Read the model definition and answer for the solid it produces. Units are mm, in the model's axes. A direction names the side the tool comes from. Coordinates: 2 decimals unless noted, no trailing zeros. Write each loop counter-clockwise with the first axis right and the second up, starting at its lowest first coordinate (ties: lowest second). Pieces come first, ordered by that corner, then holes.
1) Find the intervals of material crossed by line 1 (Z direction, x = 1774, y = -566.25) (3 decimals); line 2 (Y direction, x = 1786.7, z = 694.25) (3 decimals); line 3 (Z direction, x = 1767.5, y = -562.5) (3 decimals), in increasing order.
2) The part is cut by section A-A (x = 1786.7). Give the number of separate pieces and of enclosed holes in the cut face, then the cut area to 3 significant figures.
3) Each of these flat-tipped pins is pushed along its axis until it touches: pin 1 Ø2 at (x, z) = (1804.5, 580.5) entering from +Y (3 decimals); pin 2 Ø8 at (x, y) = (1775.5, -475.5) entering from -Z (3 decimals); pin 3 Ø11.5 at (x, y) = (1786.7, -480.185) entering from +Z (3 decimals). Where does it stop, or does it pass through?
4) The part is cut by section C-C (z = 425.5). Determine the outline of the cut face in (x, y) (3 decimals).
5) The part is cut by section B-B (y = -457). Determine the outline of the cut face in (x, z) (3 decimals), then the cut area to 3 significant figures.
6) Which of the six approach directions +Z, -Z, +X, -X, +Y, -Y give full straight-line access (tool end or side, diameter ignored) to faces 1 (the face through (1787, -564.085, 500)), 2 (the face through (1784.01, -475.97, 693.12))?
7) Determine the mould class of faces 3 (the face through (1812.1, -568, 501)), 4 (the face through (1782.475, -567.196, 547.743)), 5 (the face through (1787, -507, 696.315)) for opening direction X: +X half, -X half, draft (parallel to the pull), parting line (faces both ways), or undercut.
from build123d import *

# Parameters (mm, degrees)
CROQUIS2_W              = 50.8
CROQUIS2_H              = 6.31
CROQUIS3_W              = 50.8
CROQUIS3_H              = 6.31
CROQUIS4_W              = 60
CROQUIS4_H              = 53.155
SALIENTE_EXTRUIR1_DEPTH = 6.31
CROQUIS5_W              = 60
CROQUIS5_H              = 6.31
CORTAR_EXTRUIR1_DEPTH   = 6.31
CORTAR_EXTRUIR2_DEPTH   = 634
CROQUIS8_W              = 50.8
CROQUIS8_H              = 6.31
SALIENTE_EXTRUIR2_DEPTH = 63.5
CROQUIS9_R              = 5
CORTAR_EXTRUIR3_DEPTH   = 10
CROQUIS10_W             = 790.847933
CROQUIS10_H             = 6.31
CORTAR_EXTRUIR4_DEPTH   = 286
CROQUIS11_W             = 50.8
CROQUIS11_H             = 6.31
CROQUIS11_W_2           = 210
CORTAR_EXTRUIR5_DEPTH   = 13.11
CROQUIS12_W             = 50.8
CROQUIS12_H             = 6.31
SALIENTE_EXTRUIR3_DEPTH = 6.35
CROQUIS13_W             = 50.8
CROQUIS13_H             = 6.35
CORTAR_EXTRUIR6_DEPTH   = 6.35
CROQUIS14_W             = 85.847108528
CROQUIS14_H             = 473.639219469
CORTAR_EXTRUIR7_DEPTH   = 137
CROQUIS15_R             = 4.7625
CORTAR_EXTRUIR8_DEPTH   = 33
CROQUIS16_R             = 5
CORTAR_EXTRUIR9_DEPTH   = 33
CROQUIS18_R             = 4.7625
CORTAR_EXTRUIR10_DEPTH  = 50


with BuildPart() as part:
    # Barrer1: sweep along a curve in space
    with BuildLine() as barrer1_path:
        Line((0, 0, 0), (0, -567.24, 0))
        Line((0, -567.24, 0), (0, -567.24, 336.2))
        Line((0, -567.24, 336.2), (1786.7, -567.24, 336.2))
        Line((1786.7, -567.24, 336.2), (1786.7, -567.24, 693.16))
        Line((1786.7, -567.24, 693.16), (1786.7, -436.23, 693.16))
        Line((1786.7, -436.23, 693.16), (1786.7, -436.23, 1487.162933))
    # Croquis2 → Barrer1 (sweep)
    with BuildSketch(Plane(origin=(0, 0, 0), x_dir=(1, 0, 0), z_dir=(0, 1, 0))):
        Rectangle(CROQUIS2_W, CROQUIS2_H)
        with Locations((210, 0)):
            Rectangle(CROQUIS2_W, CROQUIS2_H)
    sweep(path=barrer1_path.line, transition=Transition.RIGHT)

    # Barrer4: sweep along a curve in space
    with BuildLine() as barrer4_path:
        Line((-0.201028049, -3.155, -3.155), (-0.201028049, -3.155, -207.155))
        Line((-0.201028049, -3.155, -207.155), (-0.201028049, -53.155, -207.155))
    # Croquis3 → Barrer4 (sweep)
    with BuildSketch(Plane(origin=(0, 0, -3.155), x_dir=(-1, 0, 0), z_dir=(0, 0, -1))):
        with Locations((-210, -3.155)):
            Rectangle(CROQUIS3_W, CROQUIS3_H)
        with Locations((0, -3.155)):
            Rectangle(CROQUIS3_W, CROQUIS3_H)
    sweep(path=barrer4_path.line, transition=Transition.RIGHT)

    # Croquis4 → Saliente-Extruir1 (add)
    with BuildSketch(Plane(origin=(0, 0, -210.31), x_dir=(-1, 0, 0), z_dir=(0, 0, -1))):
        with Locations((-154.6, -26.5775)):
            Rectangle(CROQUIS4_W, CROQUIS4_H)
    extrude(amount=-SALIENTE_EXTRUIR1_DEPTH)

    # Croquis5 → Cortar-Extruir1 (cut)
    with BuildSketch(Plane.XY.offset(-204)):
        with Locations((154.6, -3.155)):
            Rectangle(CROQUIS5_W, CROQUIS5_H)
    extrude(amount=-CORTAR_EXTRUIR1_DEPTH, mode=Mode.SUBTRACT)

    # Croquis7 → Cortar-Extruir2 (cut)
    with BuildSketch(Plane(origin=(0, 0, 0), x_dir=(1, 0, 0), z_dir=(0, 1, 0))):
        Polygon((1761.3, -361.6), (2022.1, -361.6), (2022.1, 278.600557529), (-188.115947115, 278.600557529), (-188.115947115, -361.6), align=None)
    extrude(amount=-CORTAR_EXTRUIR2_DEPTH, mode=Mode.SUBTRACT)

    # Croquis8 → Saliente-Extruir2 (add)
    with BuildSketch(Plane(origin=(0, 0, 361.6), x_dir=(-1, 0, 0), z_dir=(0, 0, -1))):
        with Locations((-1786.7, -567.24)):
            Rectangle(CROQUIS8_W, CROQUIS8_H)
    extrude(amount=SALIENTE_EXTRUIR2_DEPTH)

    # Croquis9 → Cortar-Extruir3 (cut)
    with BuildSketch(Plane(origin=(0, -433.075, 0), x_dir=(1, 0, 0), z_dir=(0, 1, 0))):
        with Locations(Location((1786.7, -1454.162933, 0), (0, 0, 270))):
            Circle(CROQUIS9_R)
        with Locations(Location((1786.7, -1234.162933, 0), (0, 0, 270))):
            Circle(CROQUIS9_R)
        with Locations(Location((1996.7, -1234.162933, 0), (0, 0, 270))):
            Circle(CROQUIS9_R)
        with Locations(Location((1996.7, -1454.162933, 0), (0, 0, 270))):
            Circle(CROQUIS9_R)
    extrude(amount=-CORTAR_EXTRUIR3_DEPTH, mode=Mode.SUBTRACT)

    # Croquis10 → Cortar-Extruir4 (cut)
    with BuildSketch(Plane(origin=(2022.1, 0, 0), x_dir=(0, 0, -1), z_dir=(1, 0, 0))):
        with Locations((-1091.7389665, -436.23)):
            Rectangle(CROQUIS10_W, CROQUIS10_H)
    extrude(amount=-CORTAR_EXTRUIR4_DEPTH, mode=Mode.SUBTRACT)

    # Croquis11 → Cortar-Extruir5 (cut)
    with BuildSketch(Plane(origin=(0, -433.075, 0), x_dir=(1, 0, 0), z_dir=(0, 1, 0))):
        with Locations((1996.7, -693.16)):
            Rectangle(CROQUIS11_W, CROQUIS11_H)
        with Locations((1866.3, -693.16)):
            Rectangle(CROQUIS11_W_2, CROQUIS11_H)
    extrude(amount=-CORTAR_EXTRUIR5_DEPTH, mode=Mode.SUBTRACT)

    # Croquis12 → Saliente-Extruir3 (add)
    with BuildSketch(Plane(origin=(0, 0, 361.6), x_dir=(-1, 0, 0), z_dir=(0, 0, -1))):
        with Locations((-1996.7, -567.24)):
            Rectangle(CROQUIS12_W, CROQUIS12_H)
    extrude(amount=SALIENTE_EXTRUIR3_DEPTH)

    # Croquis13 → Cortar-Extruir6 (cut)
    with BuildSketch(Plane(origin=(0, -564.085, 0), x_dir=(1, 0, 0), z_dir=(0, 1, 0))):
        with Locations((1786.7, -301.275)):
            Rectangle(CROQUIS13_W, CROQUIS13_H)
    extrude(amount=-CORTAR_EXTRUIR6_DEPTH, mode=Mode.SUBTRACT)

    # Croquis14 → Cortar-Extruir7 (cut)
    with BuildSketch(Plane(origin=(0, -446.185, 0), x_dir=(1, 0, 0), z_dir=(0, 1, 0))):
        with Locations((1999.254154868, -571.717300183)):
            Rectangle(CROQUIS14_W, CROQUIS14_H)
    extrude(amount=-CORTAR_EXTRUIR7_DEPTH, mode=Mode.SUBTRACT)

    # Croquis15 → Cortar-Extruir8 (cut)
    with BuildSketch(Plane(origin=(0, -564.085, 0), x_dir=(1, 0, 0), z_dir=(0, 1, 0))):
        with Locations(Location((1786.7, -545.545, 0), (0, 0, 270))):
            Circle(CROQUIS15_R)
    extrude(amount=-CORTAR_EXTRUIR8_DEPTH, mode=Mode.SUBTRACT)

    # Croquis16 → Cortar-Extruir9 (cut)
    with BuildSketch(Plane(origin=(0, 0, 690.005), x_dir=(-1, 0, 0), z_dir=(0, 0, -1))):
        with Locations((-1786.7, -480.185)):
            Circle(CROQUIS16_R)
    extrude(amount=-CORTAR_EXTRUIR9_DEPTH, mode=Mode.SUBTRACT)

    # Croquis18 → Cortar-Extruir10 (cut)
    with BuildSketch(Plane(origin=(0, -570.395, 0), x_dir=(-1, 0, 0), z_dir=(0, -1, 0))):
        with Locations(Location((-1799.399999999, -342.552204666, 0), (0, 0, 90))):
            Circle(CROQUIS18_R)
        with Locations(Location((-1773.999999999, -317.152204666, 0), (0, 0, 90))):
            Circle(CROQUIS18_R)
    extrude(amount=-CORTAR_EXTRUIR10_DEPTH, mode=Mode.SUBTRACT)


solid = part.part
Reported:
1. line 1: z = 304.45 to 312.39, 321.915 to 696.315
1. line 2: y = -570.395 to -485.185, -475.185 to -446.185
1. line 3: z = 690.005 to 696.315
2. separate pieces: 3
2. enclosed holes: 0
2. area: 3,090 mm2
3. pin 1: stops at y = -564.085
3. pin 2: stops at z = 690.005
3. pin 3: stops at z = 696.315
4. outline: (1761.3, -570.395) - (1812.1, -570.395) - (1812.1, -564.085) - (1761.3, -564.085) - close
5. outline: (1761.3, 690.005) - (1812.1, 690.005) - (1812.1, 696.315) - (1761.3, 696.315) - close
5. area: 321 mm2
6. face 1: -Z, +X, -X, +Y
6. face 2: +Z, -Z
7. face 3: +X half
7. face 4: undercut
7. face 5: draft
